```python
from build123d import *

# Parameters (mm, degrees)
SKETCH1_R           = 30
SKETCH1_R_2         = 5
BOSS_EXTRUDE1_DEPTH = 50
SKETCH2_W           = 25
SKETCH2_H           = 30
CUT_EXTRUDE1_DEPTH  = 101


with BuildPart() as part:
    # Sketch1 → Boss-Extrude1 (new body)
    with BuildSketch(Plane(origin=(0, 0, 0), x_dir=(1, 0, 0), z_dir=(0, 1, 0))):
        with BuildLine():
            Line((-50, -60), (-50, 0))
            ThreePointArc((-50, 0), (0, 50), (50, 0))
            Line((50, 0), (50, -60))
            Line((50, -60), (50, -100))
            ThreePointArc((50, -100), (47.071067812, -107.071067812), (40, -110))
            Line((40, -110), (-40, -110))
            ThreePointArc((-40, -110), (-47.071067812, -107.071067812), (-50, -100))
            Line((-50, -100), (-50, -60))
        make_face()
        Circle(SKETCH1_R, mode=Mode.SUBTRACT)
        with Locations((-15, -100)):
            Circle(SKETCH1_R_2, mode=Mode.SUBTRACT)
        with Locations((15, -100)):
            Circle(SKETCH1_R_2, mode=Mode.SUBTRACT)
    extrude(amount=BOSS_EXTRUDE1_DEPTH)

    # Sketch2 → Cut-Extrude1 (cut, through all)
    with BuildSketch(Plane(origin=(50, 0, 0), x_dir=(0, 0, -1), z_dir=(1, 0, 0))):
        with Locations((-97.5, 25)):
            Rectangle(SKETCH2_W, SKETCH2_H)
    extrude(amount=-CUT_EXTRUDE1_DEPTH, mode=Mode.SUBTRACT)


solid = part.part
```
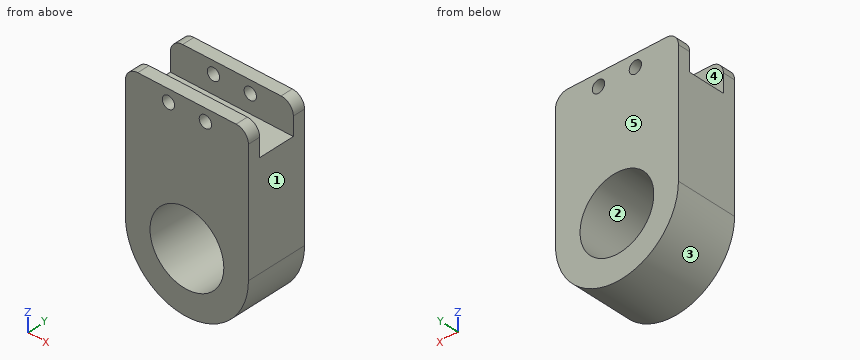
Part model, mm, in its own coordinate system. Face numbers are marked on the shaded views. A direction names the side the tool comes from. Give positions to 0.01 mm unless a question says otherwise; leave off trailing zeros. Loops run counter-clockwise (first coordinate to the right, second up) from the corner with the lowest first, then second, coordinate; pieces in that order, holes last. Notation, with made-up numbers: M 0,22.5 L 10,22.5 A27 ccw 10,59.5 Z; hole C -15,85 d10. An arc over 180 degrees is marked long. Return JSON: item names as keys, results as strings.
1) Saw through at A-A, the plane z = -26.5. List the corners of the cut face in (x, y).
Calculated:
{"outline": "M -42.4,0 L -14.06,0 L -14.06,50 L -42.4,50 Z; M 14.06,0 L 42.4,0 L 42.4,50 L 14.06,50 Z"}
2) Saw through at C-C, the plane x = -15. List the corners of the cut face in (y, z), then the cut area to 3 significant figures.
Calculated:
{"outline": "M 0,-47.7 L 50,-47.7 L 50,-25.98 L 0,-25.98 Z; M 0,25.98 L 50,25.98 L 50,95 L 40,95 L 40,85 L 10,85 L 10,95 L 0,95 Z; M 0,105 L 10,105 L 10,110 L 0,110 Z; M 40,105 L 50,105 L 50,110 L 40,110 Z", "area": "4,340 mm2"}
3) Saw through at B-B, the plane y = 44. List the corners of the cut face in (x, z).
Calculated:
{"outline": "M -50,0 A50 ccw 50,0 L 50,100 A10 ccw 40,110 L -40,110 A10 ccw -50,100 Z; hole C 0,0 d60; hole C -15,100 d10; hole C 15,100 d10"}
4) Flat gauge pins, fed straight in: pin 1 Ø2 at (x, y) = (-36, 25) entering from +Z; pin 2 Ø1 at (y, z) = (11.5, -13.5) entering from +X; pin 3 Ø1.5 at (x, y) = (-38, 42) entering from -Z. Where does each tip first touch, or does it go through?
Calculated:
{"pin 1": "stops at z = 85", "pin 2": "stops at x = 48.28", "pin 3": "stops at z = -33.35"}
5) Pull direction Z, two halves, no side cores. Call the marked faces 1, 2 and 3: released by +Z, released by -Z, zero draft, split by the parting line, or undercut.
Calculated:
{"face 1": "zero draft", "face 2": "undercut", "face 3": "released by -Z"}
6) Saw through at D-D, the plane x = 25. List the corners of the cut face in (y, z).
Calculated:
{"outline": "M 0,-43.3 L 50,-43.3 L 50,-16.58 L 0,-16.58 Z; M 0,16.58 L 50,16.58 L 50,110 L 40,110 L 40,85 L 10,85 L 10,110 L 0,110 Z"}
7) Drill centre lines: line 1 (X direction, y = 4.5, z = 100); line 2 (Z direction, x = 0, y = 37.5); line 3 (Y direction, x = -8.5, z = 89). Where is each one in solid material? Low to high.
Calculated:
{"line 1": "x = -50 to -20, -10 to 10, 20 to 50", "line 2": "z = -50 to -30, 30 to 85", "line 3": "y = 0 to 10, 40 to 50"}
8) 3-axis set-ups, long thin cutter, end or side, ignore diameter. For the marked faces 4 and 5: which of +Z, -Z, +X, -X, +Y, -Y reach the whole face in a straight line?
Calculated:
{"face 4": "+Z, +X, -X", "face 5": "+Z, -Z, +X, -X, +Y"}
